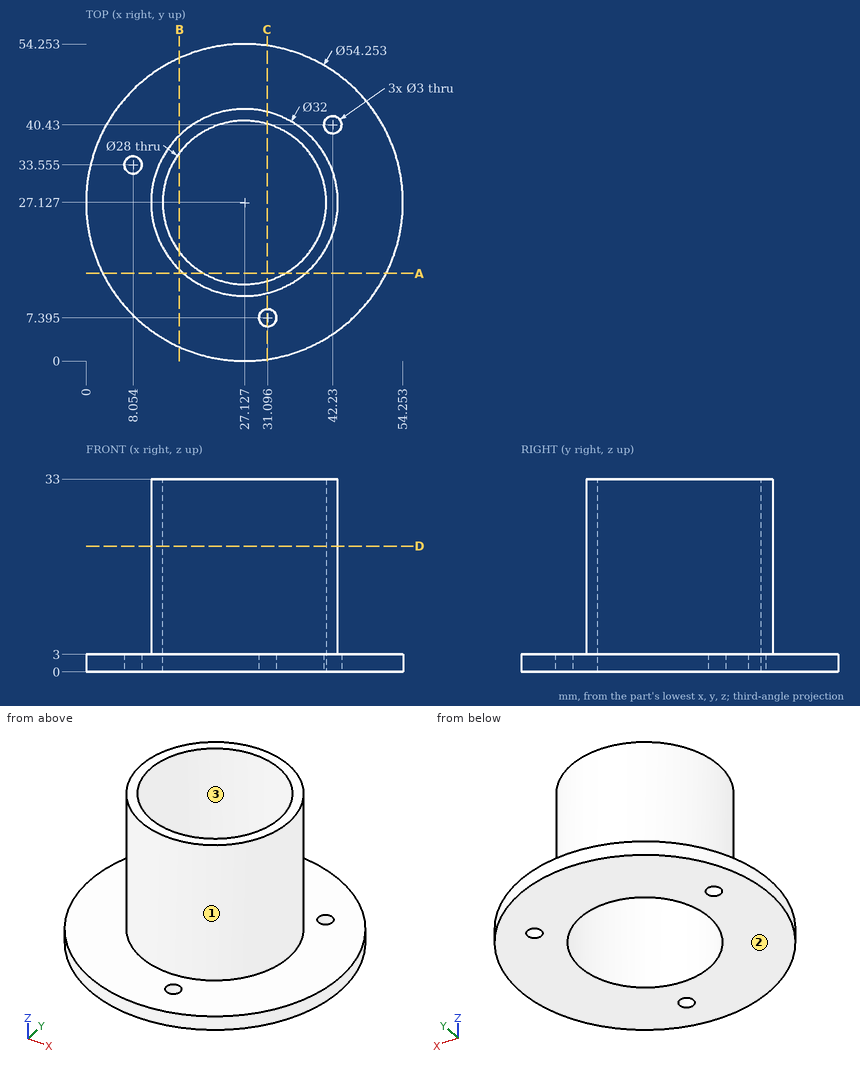
Check sheet for the drawn part. Datum: minimum x, y, z corner. Units: mm. Coordinates: 2 decimals unless noted, no trailing zeros. Loops run counter-clockwise (first coordinate to the right, second up) from the corner with the lowest first, then second, coordinate; pieces in that order, holes last. Notation, with made-up numbers: (7.5, 60) -> (40.5, 60) arc R15 ccw to (40.5, 79) -> close; hole circle Ø10 at (72.25, 29). An arc over 180 degrees is marked (long way). Answer as a JSON object with one key per item and string values. Group by question number.
Item 1: Sectioned sample at B-B on x = 16. Record the boundary of the cut face in (y, z) (1 decimal).
Item 2: Scan lines: probe 1 along X at (y, z) = (27, 21.5); probe 2 along X at (y, z) = (19.5, 31) (1 decimal); probe 3 along Z at (x, y) = (51.5, 38). Record each from-to range of solid material in increasing order.
Item 3: Mould release check, pull along X, two halves, no side actions. Record for the marked faces 1, 2 and 3: +X half, -X half, draft (parallel to the pull), parting line (faces both ways), or undercut.
Item 4: Sectioned sample at C-C on x = 31. State how many separate pieces and enclosed holes the cut face has.
Item 5: Depth check by flat-ended pin: pin 1 (5 mm diameter, centred on x = 19, z = 11, fed in from +Y) (1 decimal); pin 2 (1.5 mm diameter, centred on x = 27, z = 15, fed in from -Y); pin 3 (4 mm diameter, centred on x = 42.23, y = 40.43, fed in from -Z); pin 4 (6 mm diameter, centred on x = 15, z = 21, fed in from +Y). Enter the tip coordinate at first touch or a pass-through.
Item 6: Sectioned sample at A-A on y = 15. Record the boundary of the cut face in (x, z) (1 decimal), plus the area to 3 significant figures.
Item 7: Sectioned sample at D-D on z = 21.5. Record the boundary of the cut face in (x, y).
Evaluation:
{
 "1": {"outline": "(2.4, 0) -> (18.6, 0) -> (18.6, 33) -> (15.6, 33) -> (15.6, 3) -> (2.4, 3) -> close; (35.6, 0) -> (51.9, 0) -> (51.9, 3) -> (38.6, 3) -> (38.6, 33) -> (35.6, 33) -> close"},
 "2": {"probe 1": "x = 11.13 to 13.13, 41.13 to 43.13", "probe 2": "x = 13.1 to 15.4, 38.9 to 41.2", "probe 3": "z = 0 to 3"},
 "3": {"face 1": "parting line", "face 2": "draft", "face 3": "undercut"},
 "4": {"separate pieces": "3", "enclosed holes": "0"},
 "5": {"pin 1": "stops at y = 42.1", "pin 2": "stops at y = 11.13", "pin 3": "stops at z = 0", "pin 4": "stops at y = 40.27"},
 "6": {"outline": "(2.9, 0) -> (20.1, 0) -> (20.1, 33) -> (16.7, 33) -> (16.7, 3) -> (2.9, 3) -> close; (34.1, 0) -> (51.4, 0) -> (51.4, 3) -> (37.6, 3) -> (37.6, 33) -> (34.1, 33) -> close", "area": "310 mm²"},
 "7": {"outline": "circle Ø32 at (27.13, 27.13); hole circle Ø28 at (27.13, 27.13)"}
}
